from build123d import *

# Parameters (mm, degrees)
F0_R     = 20.25
F1_DEPTH = 22.5
F6_SIZE  = 2


with BuildPart() as f1:
    # F0 (on Top) → F1 (new body)
    with BuildSketch(Plane.XY):
        Polygon((30.385918036, -26.6463753341), (38.2693969761, 12.9917892694), (7.8834789401, 39.6381646035), (-30.385918036, 26.6463753341), (-38.2693969761, -12.9917892694), (-7.8834789401, -39.6381646035), align=None)
        Circle(F0_R, mode=Mode.SUBTRACT)
    extrude(amount=F1_DEPTH)

    # F4 (on 3pt) → F5 (revolve, cut)
    with BuildSketch(Plane(origin=(0, 0, 0), x_dir=(0.9469219991, 0.3214634157, 0), z_dir=(0.3214634157, -0.9469219991, 0))):
        Polygon((35, 22.707875818), (35, 22.5), (44.6592582629, 19.911809549), (44.6592582629, 22.707875818), align=None)
        Polygon((44.6592582629, 2.588190451), (35, 0), (35, -0.207875818), (44.6592582629, -0.207875818), align=None)
    revolve(axis=Axis((0, 0, 0), (0, 0, -1)), mode=Mode.SUBTRACT)

    # F6
    f6_edges = [f1.edges().sort_by_distance(p)[0] for p in [
        (-20.25, 0, 22.5),
        (-20.25, 0, 0),
    ]]
    chamfer(f6_edges, length=F6_SIZE)


solid = f1.part
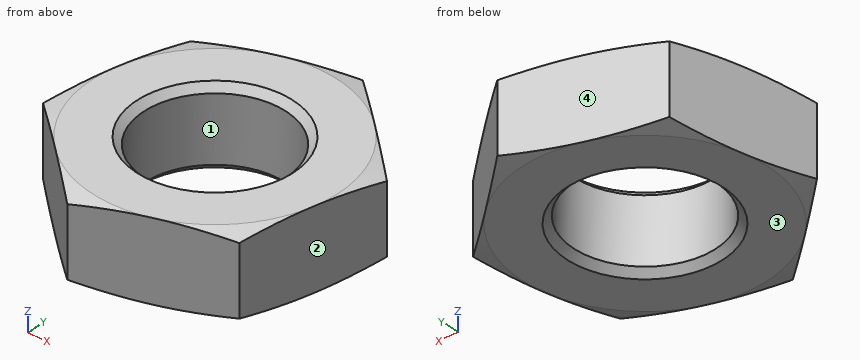
Can you work these out from the model? Positions are in its coordinate system, mm. Face numbers are marked on the shaded views. Coordinates: 2 decimals unless noted, no trailing zeros. Write each loop counter-clockwise with the first axis right and the second up, starting at its lowest first coordinate (ties: lowest second). Pieces come first, ordered by that corner, then holes.
Q1. If we mould it in two halves opening along Y, with no side actions, what happens to the marked faces 1, 2, 3 and 4? For each: +Y half, -Y half, draft (parallel to the pull), parting line (faces both ways), or undercut.
Results found:
face 1: undercut
face 2: -Y half
face 3: draft
face 4: +Y half
Q2. Imagine slicing it at C-C, the plane y = 0. List the corners of the cut face in (x, z) for me.
Results found:
outline: (-35.69, 0.18) - (-35, 0) - (-22.25, 0) - (-20.25, 2) - (-20.25, 20.5) - (-22.25, 22.5) - (-35, 22.5) - (-35.69, 22.32) - close; (20.25, 2) - (22.25, 0) - (35, 0) - (35.69, 0.18) - (35.69, 22.32) - (35, 22.5) - (22.25, 22.5) - (20.25, 20.5) - close
Q3. For P1, Ø1.5, axis at x = 14, z = 3, coming from the +Y side; P2, Ø4, axis at y = -30.5, z = 14, coming from the -X side; P3, Ø10, axis at y = -5.5, z = 13, coming from the +X side, each with a flat end and sliding along its axis, tell me the tip position at first contact or that it passes through.
Results found:
P1: stops at y = 34.93
P2: stops at x = -20.58
P3: stops at x = 35.59
Q4. Imagine slicing it at B-B, the plane x = 0. List the corners of the cut face in (y, z) for me, plus the area to 3 significant figures.
Results found:
outline: (-36.96, 0.53) - (-35, 0) - (-22.25, 0) - (-20.25, 2) - (-20.25, 20.5) - (-22.25, 22.5) - (-35, 22.5) - (-36.96, 21.97) - close; (20.25, 2) - (22.25, 0) - (35, 0) - (36.96, 0.53) - (36.96, 21.97) - (35, 22.5) - (22.25, 22.5) - (20.25, 20.5) - close
area: 742 mm2
Q5. Please list where these lines run through material, in increasing order: L1, parallel to Y at x = 0, z = 15.5; L2, parallel to X at y = -10, z = 1.75; L3, parallel to Z at x = 8.5, y = 19.
Results found:
L1: y = -36.96 to -20.25, 20.25 to 36.96
L2: x = -37.67 to -17.9, 17.9 to 33.7
L3: z = 1.44 to 21.06
Q6. Imagine slicing it at A-A, the plane z = 8.25. List the corners of the cut face in (x, y) for me, plus the area to 3 significant figures.
Results found:
outline: (-38.27, -12.99) - (-7.88, -39.64) - (30.39, -26.65) - (38.27, 12.99) - (7.88, 39.64) - (-30.39, 26.65) - close; hole circle Ø40.5 at (0, 0)
area: 2,960 mm2
